Design review of the part built by this model. Coordinates are the model's own, in mm. A direction names the side the tool comes from. Round coordinates to 2 decimals unless told otherwise and drop trailing zeros. Order: outer loops, then holes, each group sorted by start corner. A loop starts at its lowest first (then second) coordinate and runs counter-clockwise, first axis right, second up. Notation, with made-up numbers: M 61,63 L 68,63 A28 cw 68,96 Z; hole C 23.25,-22 d6. An arc over 180 degrees is marked long. Write item = value, one per line. Start each with the question number.
```python
from build123d import *

# Parameters (mm, degrees)
F0_W     = 50.8
F0_H     = 38.1
F1_DEPTH = 127
F2_R     = 12.7
F3_R     = 12.7
F4_DEPTH = 25.4
F5_R     = 17.78
F6_DEPTH = 25.4


with BuildPart() as f1:
    # F0 (on Right) → F1 (new body)
    with BuildSketch(Plane.YZ):
        with Locations((-22.797512, 19.314706)):
            Rectangle(F0_W, F0_H)
    extrude(amount=F1_DEPTH)

    # F2
    f2_edges = [f1.edges().sort_by_distance(p)[0] for p in [
        (63.5, -48.197512, 38.364706),
        (63.5, 2.602488, 38.364706),
        (63.5, -48.197512, 0.264706),
        (63.5, 2.602488, 0.264706),
    ]]
    fillet(f2_edges, radius=F2_R)

    # F3 (on face) → F4 (cut)
    with BuildSketch(Plane(origin=(0, 0, 0.264706), x_dir=(1, 0, 0), z_dir=(0, 0, -1))):
        with Locations((92.420697, 22.85873)):
            Circle(F3_R)
    extrude(amount=-F4_DEPTH, mode=Mode.SUBTRACT)

    # F5 (on face) → F6 (join)
    with BuildSketch(Plane.YZ.offset(127)):
        with Locations((-22.503506, 19.241814)):
            Circle(F5_R)
    extrude(amount=F6_DEPTH)


solid = f1.part
```
(1) For faces 5 (the face through (127, -40, 24)), 6 (the face through (63, 2.602, 19)), 7 (the face through (104.15, -17.99, 12.79)), list the 3-axis set-ups (+Z, -Z, +X, -X, +Y, -Y) from which the entire face can be reached by the end or side of a thin tool; tool diameter is ignored.
(2) Consider section C-C, the plane y = -21. Write out the cut boundary in (x, z).
(3) Draft analysis for pull direction Y (two halves, no side actions). For faces 1 (the face through (64.389, -44.576, 4.084)), 2 (the face through (139.52, -6.08, 12.43)), 3 (the face through (63, -23, 38.365)), 4 (the face through (92, -23, 25.665)), state which applies: pulls with the +Y half, pulls with the -Y half, needs draft (parallel to the pull), parting line crosses it, or undercut.
(4) Insertion check: pin 1 (1 mm diameter, centred on x = 124.5, z = 10.5, fed in from +Y); pin 2 (1.5 mm diameter, centred on x = 65.5, z = 12, fed in from +Y); pin 3 (12.5 mm diameter, centred on x = 95.5, y = -18.5, fed in from -Z). Each pin has a flat end and moves straight along its axis. Give the tip position at first contact, or say it passes through.
(5) For line 1 along X through (y, z) = (-22, 9.5); line 2 along X through (y, z) = (-2, 26.5); line 3 along Z through (x, y) = (98.5, -13), list the stretches that pass through material, from the lowest coordinate up. Write a range as [from, to].
(6) Consider section D-D, the plane z = 30.5. Write out the cut boundary in (x, y), then the cut area to 3 significant figures.
(7) Consider section B-B, the plane x = 108.5. Write out the cut boundary in (y, z), then the cut area to 3 significant figures.
(8) Consider section A-A, the plane z = 7. Write out the cut boundary in (x, y).
Completed:
q1.face_5 = +X
q1.face_6 = +Z, -Z, +X, -X, +Y
q1.face_7 = -Z
q2.outline = M 0,0.26 L 79.86,0.26 L 79.86,25.66 L 104.98,25.66 L 104.98,0.26 L 127,0.26 L 127,1.53 L 152.4,1.53 L 152.4,36.96 L 127,36.96 L 127,38.36 L 0,38.36 Z
q3.face_1 = pulls with the -Y half
q3.face_2 = parting line crosses it
q3.face_3 = needs draft
q3.face_4 = undercut
q4.pin_1 = 2.45
q4.pin_2 = 2.6
q4.pin_3 = 25.66
q5.line_1 = [0, 79.75], [105.09, 152.4]
q5.line_2 = [0, 127]
q5.line_3 = [25.66, 38.36]
q6.outline = M 0,-47.24 L 127,-47.24 L 127,-36.27 L 152.4,-36.27 L 152.4,-8.74 L 127,-8.74 L 127,1.65 L 0,1.65 Z
q6.area = 6,910 mm2
q7.outline = M -48.2,12.96 A12.7 ccw -35.5,0.26 L -10.1,0.26 A12.7 ccw 2.6,12.96 L 2.6,25.66 A12.7 ccw -10.1,38.36 L -35.5,38.36 A12.7 ccw -48.2,25.66 Z
q7.area = 1,800 mm2
q8.outline = M 0,-46.71 L 127,-46.71 L 127,-35.4 L 152.4,-35.4 L 152.4,-9.61 L 127,-9.61 L 127,1.11 L 0,1.11 Z; hole C 92.42,-22.86 d25.4
